Can you work these out from the model? Positions are in its coordinate system, mm. Face numbers are marked on the shaded views. Round coordinates to 2 decimals unless told otherwise and drop trailing zeros. Order: outer loops, then holes, each group sorted by start corner. A loop starts at its lowest first (then second) coordinate and runs counter-clockwise, first axis right, second up.
Q1. If we section it at A-A (y = 0): Please give me the cut outline in (x, z).
Q2. If we section it at D-D (x = 7): Please give me the cut outline in (y, z), plus the area to 3 significant figures.
Q3. We'd pull the mould along Z, two halves only. Please class the marked faces 1, 2 and 3: pulls with the +Z half, pulls with the -Z half, needs draft (parallel to the pull), parting line crosses it, or undercut.
Q4. If I drill on line 1 (Y direction, x = 0, z = 0.1); line 2 (X direction, y = 0.25, z = 0.25), over which ranges is the centre line in solid material (lowest first)?
Q5. If we section it at C-C (z = 3.4): Please give me the cut outline in (x, y), plus the area to 3 significant figures.
Q6. Will these pins go through, and if not, where does the flat tip stop? P1, Ø1, axis at x = 5, z = 1, coming from the -Y side; P2, Ø1, axis at x = -4, z = 1.5, coming from the +Y side.
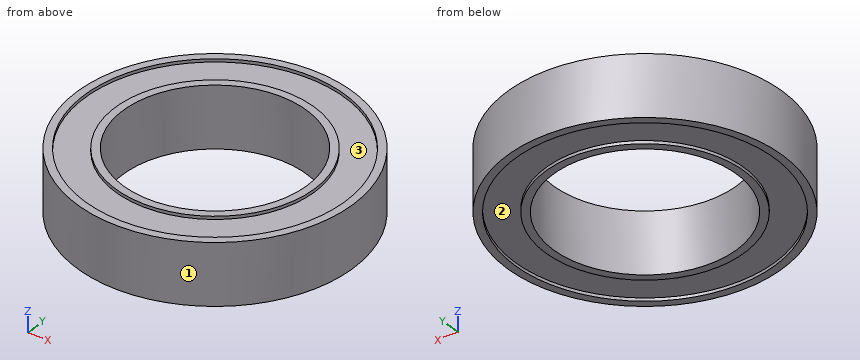
Autodesk Inventor part; units mm, degrees
ref_plane "Work Plane1" through (0, 0, 0.2) normal (0, 0, 1) x (1, 0, 0)
ref_plane "YZ Plane" through (0, 0, 0) normal (1, 0, 0) x (0, 1, 0)
ref_plane "XZ Plane" through (0, 0, 0) normal (0, 1, 0) x (-1, 0, 0)
sketch "Sketch1" plane through (0, 0, 0) normal (0, 0, 1) x (1, 0, 0)
  circle A0 centre (0, 0) radius 9
  circle A1 centre (0, 0) radius 6
  circle A2 centre (0, 0) radius 6.5
  circle A3 centre (0, 0) radius 8.5
  dimension "d0" = 18
  dimension "d1" = 12
  dimension "d2" = 0.5
  dimension "d3" = 0.5
extrude "Extrusion1" add sketch "Sketch1" along normal blind 4
ref_plane "Work Plane1" through (0, 0, 0.2) normal (0, 0, 1) x (1, 0, 0)
sketch "Sketch2" plane through (0, 0, 0.2) normal (0, 0, 1) x (1, 0, 0)
  circle A0 centre (0, 0) radius 8.5
  circle A1 centre (0, 0) radius 9
  circle A2 centre (0, 0) radius 6
  circle A3 centre (0, 0) radius 6.5
extrude "Extrusion2" add sketch "Sketch2" along normal blind 3.6 contours A0
properties part number "18x12x4 bearing"
Solution:
1. outline: (-9, 0) - (-8.5, 0) - (-8.5, 0.2) - (-6.5, 0.2) - (-6.5, 0) - (-6, 0) - (-6, 4) - (-6.5, 4) - (-6.5, 3.8) - (-8.5, 3.8) - (-8.5, 4) - (-9, 4) - close; (6, 0) - (6.5, 0) - (6.5, 0.2) - (8.5, 0.2) - (8.5, 0) - (9, 0) - (9, 4) - (8.5, 4) - (8.5, 3.8) - (6.5, 3.8) - (6.5, 4) - (6, 4) - close
2. outline: (-5.66, 0) - (-4.82, 0) - (-4.82, 0.2) - (4.82, 0.2) - (4.82, 0) - (5.66, 0) - (5.66, 4) - (4.82, 4) - (4.82, 3.8) - (-4.82, 3.8) - (-4.82, 4) - (-5.66, 4) - close
2. area: 41.4 mm2
3. face 1: needs draft
3. face 2: pulls with the -Z half
3. face 3: pulls with the +Z half
4. line 1: y = -9 to -8.5, -6.5 to -6, 6 to 6.5, 8.5 to 9
4. line 2: x = -9 to -5.99, 5.99 to 9
5. outline: circle Ø18 at (0, 0); hole circle Ø12 at (0, 0)
5. area: 141 mm2
6. P1: stops at y = -7.79
6. P2: stops at y = 8.29
